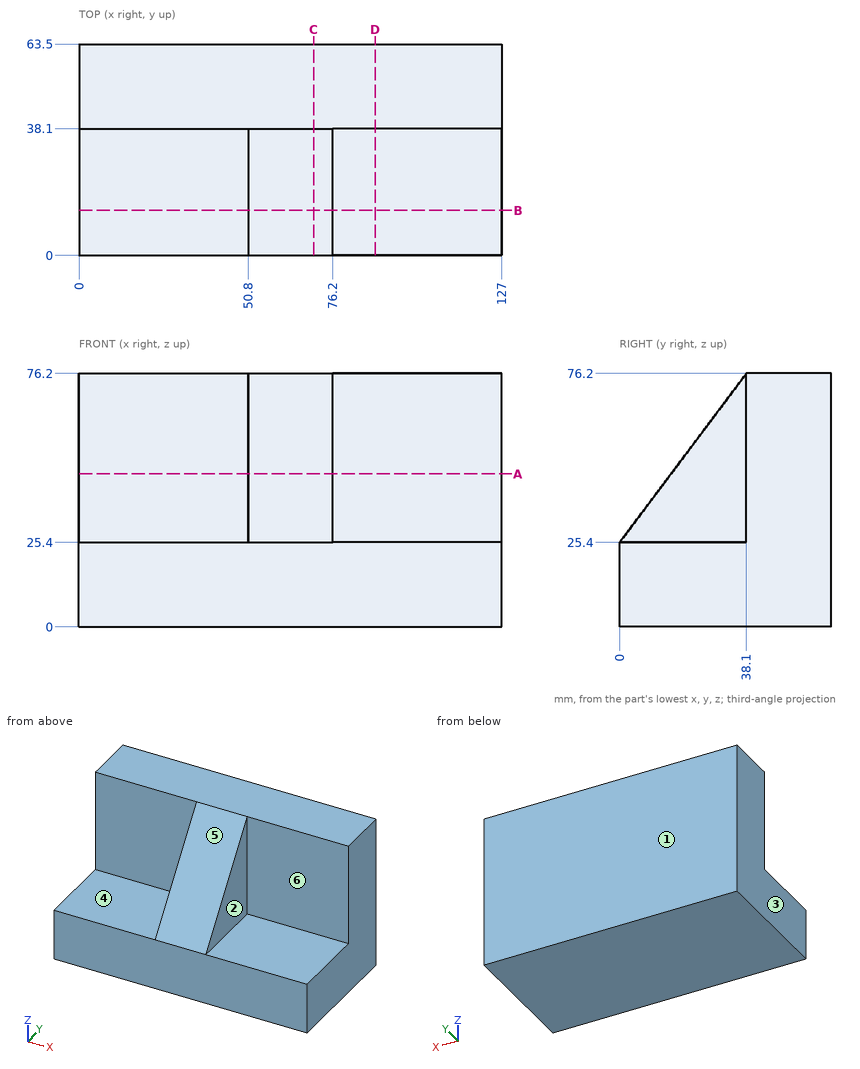
Check sheet for the drawn part. Datum: minimum x, y, z corner. Units: mm. A direction names the side the tool comes from. Coordinates: 2 decimals unless noted, no trailing zeros. Order: outer loops, then holes, each group sorted by start corner. A loop starts at its lowest first (then second) coordinate and runs counter-clockwise, first axis right, second up. Notation, with made-up numbers: M -34,84 L -9,84 A11 cw -9,98 Z; hole C 4.25,58 d7. An arc over 180 degrees is marked long. One line per question, with ' | ' between items. Start each with the question number.
Item 1: Access from +Z, -Z, +X, -X, +Y, -Y to the whole of each face (thin tool, end or side, straight path). Record for the marked faces 4, 5 and 6.
Item 2: Sectioned sample at C-C on x = 70.5. Record the cut outline in (y, z), and give its area (3 significant figures).
Item 3: Sectioned sample at A-A on z = 46. Record the cut outline in (x, y), and give its area (3 significant figures).
Item 4: Mould release check, pull along X, two halves, no side actions. Record for the marked faces 1, 2 and 3: pulls with the +X half, pulls with the -X half, needs draft (parallel to the pull), parting line crosses it, or undercut.
Item 5: Sectioned sample at B-B on y = 13.5. Record the cut outline in (x, z), and give its area (3 significant figures).
Item 6: Sectioned sample at D-D on x = 89. Record the cut outline in (y, z).
Item 7: Gauge pin test, flat ends, axial feed: P1, Ø11.5, axis at y = 14, z = 50.5, coming from the +X side; P2, Ø4, axis at x = 57, z = 66, coming from the -Y side; P3, Ø11.5, axis at x = 27.5, y = 24.5, coming from the +Z side. Record the tip position at first contact, or that the pin passes through.
Item 8: Material ranges on line 1 (Z direction, x = 9.5, y = 17.5); line 2 (Y direction, x = 94, z = 48); line 3 (X direction, y = 17.5, z = 43.5), recorded low to high.
Answer below:
1) face 4: +Z, -X, -Y | face 5: +Z, +X, -X, -Y | face 6: +Z, +X, -Y
2) outline: M 0,0 L 63.5,0 L 63.5,76.2 L 38.1,76.2 L 0,25.4 Z | area: 3,870 mm^2
3) outline: M 0,38.1 L 50.8,38.1 L 50.8,15.45 L 76.2,15.45 L 76.2,38.1 L 127,38.1 L 127,63.5 L 0,63.5 Z | area: 3,800 mm^2
4) face 1: needs draft | face 2: pulls with the +X half | face 3: pulls with the -X half
5) outline: M 0,0 L 127,0 L 127,25.4 L 76.2,25.4 L 76.2,43.4 L 50.8,43.4 L 50.8,25.4 L 0,25.4 Z | area: 3,680 mm^2
6) outline: M 0,0 L 63.5,0 L 63.5,76.2 L 38.1,76.2 L 38.1,25.4 L 0,25.4 Z
7) P1: stops at x = 76.2 | P2: stops at y = 28.95 | P3: stops at z = 25.4
8) line 1: z = 0 to 25.4 | line 2: y = 38.1 to 63.5 | line 3: x = 50.8 to 76.2
